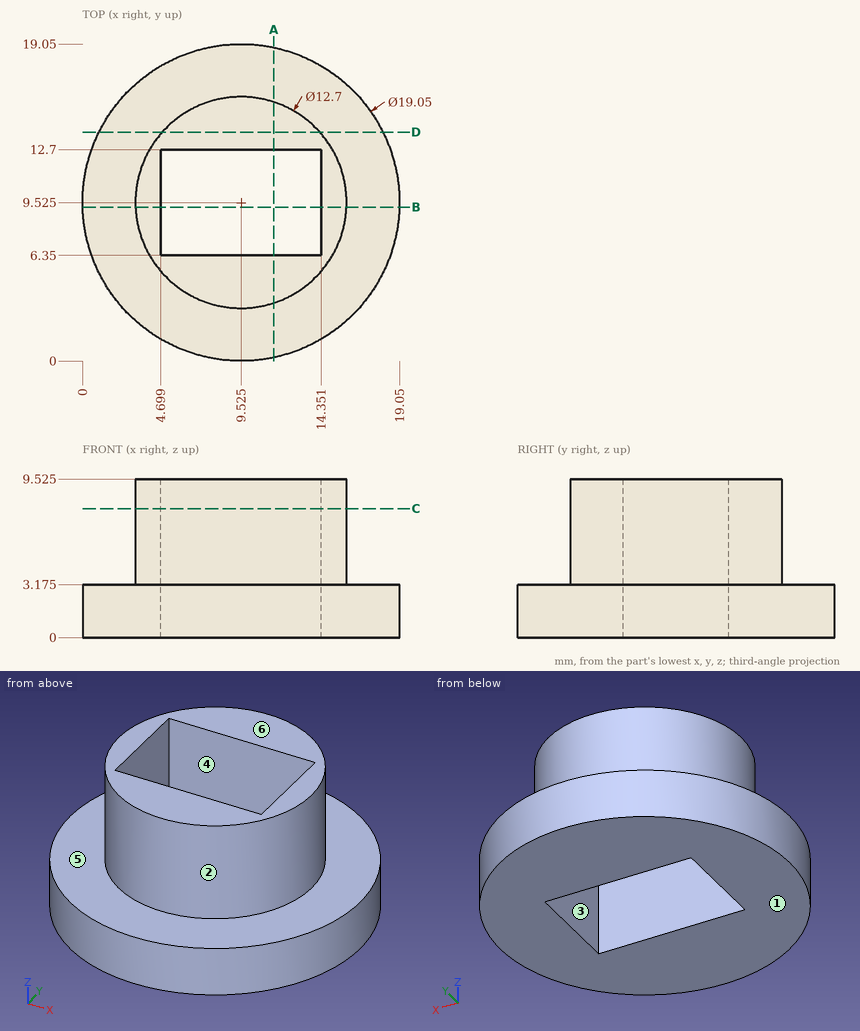
For this review, use the dimensioned drawing (mm, ordinates from the lowest corner) and the shaded views. A direction names the side the tool comes from. Coordinates: 2 decimals unless noted, no trailing zeros. Write each loop counter-clockwise with the first axis right and the second up, starting at its lowest first coordinate (ties: lowest second). Pieces come first, ordered by that corner, then holes. Notation, with made-up numbers: (61, 83.25) - (95, 83.25) arc R34 cw to (95, 113.25) - close; hole circle Ø2 at (-7, 33). An arc over 180 degrees is marked (long way). Answer in a Markdown table with one row per item. Add a question column.
Q1. Consider section D-D on y = 13.75. Give the boundary of the cut face in (x, z) (3 decimals), then the cut area to 3 significant figures.
Q2. Consider section B-B on y = 9.25. Give the boundary of the cut face in (x, z) (3 decimals).
Q3. Clearance check with flat-ended pins moving along their axes: pin 1 (5 mm diameter, centred on x = 13, z = 5, fed in from +Y); pin 2 (3 mm diameter, centred on x = 4, y = 5.5, fed in from -Z); pin 3 (3 mm diameter, centred on y = 3.5, z = 6.5, fed in from +X); pin 4 (4 mm diameter, centred on x = 14.5, z = 1, fed in from +Y). State where each tip first meets the part, or that it passes through.
Q4. To check wall thickness, follow line 1 along Y through (x, z) = (9.5, 7.25); line 2 along Z through (x, y) = (4.5, 15) (3 decimals); line 3 along X through (y, z) = (11.25, 1.25). State the ranges of each line that lie inside material, in increasing order. Write a range as from..to.
Q5. Draft analysis for pull direction X (two halves, no side actions). For the marked faces 1, 2 and 3, state which applies: +X half, -X half, draft (parallel to the pull), parting line (faces both ways), or undercut.
Q6. Consider section A-A on x = 11.5. Give the boundary of the cut face in (y, z) (3 decimals).
Q7. Consider section C-C on z = 7.75. Give the boundary of the cut face in (x, y) (3 decimals).
Q8. For the marked faces 4, 5 and 6, list the 3-axis set-ups (+Z, -Z, +X, -X, +Y, -Y) from which the entire face can be reached by the end or side of a thin tool; tool diameter is ignored.
Answers below:
| question | item | result |
|---|---|---|
| 1 | outline | (0.988, 0) - (18.062, 0) - (18.062, 3.175) - (14.265, 3.175) - (14.265, 9.525) - (4.785, 9.525) - (4.785, 3.175) - (0.988, 3.175) - close |
| 1 | area | 114 mm² |
| 2 | outline | (0.004, 0) - (4.699, 0) - (4.699, 9.525) - (3.181, 9.525) - (3.181, 3.175) - (0.004, 3.175) - close; (14.351, 0) - (19.046, 0) - (19.046, 3.175) - (15.869, 3.175) - (15.869, 9.525) - (14.351, 9.525) - close |
| 3 | pin 1 | y = 18.88 |
| 3 | pin 2 | z = 0 |
| 3 | pin 3 | x = 13.98 |
| 3 | pin 4 | y = 18.57 |
| 4 | line 1 | 3.18..6.35, 12.7..15.87 |
| 4 | line 2 | 0..3.175 |
| 4 | line 3 | 0.16..4.7, 14.35..18.89 |
| 5 | face 1 | draft |
| 5 | face 2 | parting line |
| 5 | face 3 | undercut |
| 6 | outline | (0.207, 0) - (6.35, 0) - (6.35, 9.525) - (3.49, 9.525) - (3.49, 3.175) - (0.207, 3.175) - close; (12.7, 0) - (18.843, 0) - (18.843, 3.175) - (15.56, 3.175) - (15.56, 9.525) - (12.7, 9.525) - close |
| 7 | outline | circle Ø12.7 at (9.525, 9.525); hole (4.699, 6.35) - (14.351, 6.35) - (14.351, 12.7) - (4.699, 12.7) - close |
| 8 | face 4 | +Z, -Z |
| 8 | face 5 | +Z |
| 8 | face 6 | +Z, +X, -X, +Y, -Y |
